Can you work these out from the model? Positions are in its coordinate system, mm. A direction names the side the tool comes from. Give positions to 0.01 mm unless a question says otherwise; leave off trailing zeros. Write each loop counter-clockwise with the first axis right and the second up, starting at its lowest first coordinate (ties: lowest second). Pieces come first, ordered by that corner, then holes.
Autodesk Inventor part; units mm, degrees
ref_plane "Work Plane1" through (0, 0, -15) normal (0, 0, 1) x (1, 0, 0)
ref_plane "YZ Plane" through (0, 0, 0) normal (1, 0, 0) x (0, 1, 0)
ref_plane "XZ Plane" through (0, 0, 0) normal (0, 1, 0) x (-1, 0, 0)
sketch "Sketch1" plane through (0, 0, 0) normal (0, 0, 1) x (1, 0, 0)
  line L0 (0, 0) -> (25, 0)
  line L1 (25, 0) -> (25, 40)
  line L2 (25, 40) -> (0, 40)
  line L3 (0, 40) -> (0, 0)
  dimension "d1" = 25
  dimension "d2" = 40
  dimension "d3" = 25
extrude "Extrusion1" add sketch "Sketch1" against normal blind 30
sketch "Sketch2" plane through (25, 0, 0) normal (1, 0, 0) x (0, 0, -1)
  line L0 (0, 0) -> (30, 0)
  circle A0 centre (15, 6.56) radius 2.46
extrude "Extrusion2" cut sketch "Sketch2" against normal blind 30
sketch "Sketch3" plane through (0, 0, 0) normal (-1, 0, 0) x (0, 0, 1)
  line L0 (0, 0) -> (-30, 0)
  line L1 (-25.05, 0) -> (-4.95, 0)
  line L2 (-4.95, 0) -> (-4.95, 33.12)
  line L3 (-4.95, 33.12) -> (-25.05, 33.12)
  line L4 (-25.05, 33.12) -> (-25.05, 0)
  dimension "d11" = 20.1
extrude "Extrusion3" cut sketch "Sketch3" against normal blind 20
sketch "Sketch4" plane through (0, 0, 0) normal (0, -1, 0) x (1, 0, 0)
  line L0 (20, -4.95) -> (20, -25.05)
  line L1 (20, -15) -> (25, -15)
  line L2 (25, 0) -> (25, -30)
  line L3 (20, -8.025) -> (25, -8.025)
  line L4 (25, -8.025) -> (25, -21.975)
  line L5 (25, -21.975) -> (20, -21.975)
  line L6 (20, -21.975) -> (20, -8.025)
  line L7 (20, -8.025) -> (25, -21.975) construction
  line L8 (25, -8.025) -> (20, -21.975) construction
  line L9 (25, -12.54) -> (25, -17.46)
  point P0 (0, 0)
  point P1 (22.5, -15)
  dimension "d14" = 13.95
extrude "Extrusion4" add sketch "Sketch4" along normal blind 15
sketch "Sketch5" plane through (20, 0, 0) normal (-1, 0, 0) x (0, 0, 1)
  circle A0 centre (-15, 6.56) radius 2.46
  circle A1 centre (-15, 6.56) radius 4.7025
  circle A2 centre (-15, 6.56) radius 2.46
  circle A3 centre (-15, 6.56) radius 2.46
  point P0 (0, 0)
  dimension "d17" = 9.405
extrude "Extrusion5" cut sketch "Sketch5" against normal blind 2.1
sketch "Sketch6" plane through (25, 0, 0) normal (1, 0, 0) x (0, 0, -1)
  circle A0 centre (15, 6.56) radius 4.7025
  line L0 (15, 6.56) -> (15, 23.56)
  circle A1 centre (15, 23.56) radius 2.46
  point P0 (0, 0)
  dimension "d20" = 17
  dimension "d21" = 4.92
extrude "Extrusion6" cut sketch "Sketch6" against normal blind 10 contours A1
sketch "Sketch7" plane through (20, 0, 0) normal (-1, 0, 0) x (0, 0, 1)
  circle A0 centre (-15, 23.56) radius 2.46
  circle A1 centre (-15, 23.56) radius 4.7025
  point P0 (0, 0)
  dimension "d24" = 9.405
extrude "Extrusion7" cut sketch "Sketch7" against normal blind 2.1
sketch "Sketch9" plane through (25, 0, 0) normal (1, 0, 0) x (0, 0, -1)
  circle A0 centre (15, 6.56) radius 2.46
  circle A1 centre (15, 6.56) radius 2.46
  circle A2 centre (15, 23.56) radius 2.46
  circle A3 centre (15, 23.56) radius 2.46
  line L0 (30, 40) -> (30, 0)
  line L1 (30, 0) -> (30, 40)
  line L2 (30, 40) -> (0, 40)
  line L3 (0, 40) -> (0, 0)
  line L4 (0, 0) -> (8.025, 0)
  line L5 (21.975, 0) -> (21.975, -15)
  line L6 (21.975, -15) -> (8.025, -15)
  line L7 (8.025, -15) -> (8.025, 0)
  line L8 (0, 0) -> (8.025, 0)
  line L9 (21.975, 0) -> (30, 0)
extrude "Extrusion8" add sketch "Sketch9" along normal blind 5
sketch "Sketch10" plane through (0, 40, 0) normal (0, 1, 0) x (1, 0, 0)
  line L0 (0, 30) -> (30, 30)
  line L1 (30, 0) -> (0, 0)
  line L2 (0, 30) -> (30, 30)
  line L3 (30, 30) -> (30, 0)
  line L4 (30, 0) -> (0, 0)
  line L5 (0, 0) -> (0, 30)
extrude "Extrusion9" add sketch "Sketch10" along normal blind 30
sketch "Sketch12" plane through (30, 0, 0) normal (1, 0, 0) x (0, 0, -1)
  circle A0 centre (15, 6.56) radius 2.46
  line L0 (15, 6.56) -> (15, 15.06)
  circle A1 centre (15, 15.06) radius 2.525
  point P0 (0, 0)
  dimension "d31" = 8.5
  dimension "d33" = 5.05
extrude "Extrusion10" cut sketch "Sketch12" against normal blind 30 contours A1
sketch "Sketch15" plane through (0, 0, -25.05) normal (-1, 0, 0) x (0, 0, 1)
  line L0 (0, 33.12) -> (20.1, 33.12)
  line L1 (20.1, 33.12) -> (20.1, 0)
  line L2 (0, 33.12) -> (20.1, 33.12)
  line L3 (20.1, 33.12) -> (20.1, 31.1)
  line L4 (20.1, 31.1) -> (0, 31.1)
  line L5 (0, 31.1) -> (0, 33.12)
  point P0 (25.05, 0)
  dimension "d57" = 2.02
extrude "Extrusion13" add sketch "Sketch15" against normal blind 20
sketch "Sketch17" plane through (0, 0, 0) normal (0, 0, 1) x (1, 0, 0)
  line L0 (0, 70) -> (30, 70)
  line L1 (30, 70) -> (50.0622, 90.0622)
  line L2 (30, 70) -> (80, 70) construction
  line L3 (11.9522, 97.2454) -> (0, 85.2932)
  line L4 (0, 70) -> (0, 85.2932)
  line L5 (0, 70) -> (0, 0)
  line L6 (0, 70) -> (30, 70)
  line L7 (10.923, 112.2849) -> (0, 120.567)
  line L8 (50.0622, 105.3553) -> (50.0622, 120.567)
  line L9 (50.0622, 105.3553) -> (50.0622, 90.0622)
  arc A0 (11.9522, 97.2454) -> (10.923, 112.2849) centre (4.8811, 104.3165) ccw
  line L10 (0, 150.567) -> (30, 150.567)
  line L11 (30, 150.567) -> (50.0622, 120.567)
  line L12 (5, 147.567) -> (0, 150.567)
  line L13 (5, 123.567) -> (0, 120.567)
  line L14 (5, 123.567) -> (10, 135.567)
  line L15 (10, 135.567) -> (5, 147.567)
  dimension "d61" = 45
  dimension "d62" = 32.0271
  dimension "d72" = 10
extrude "Extrusion14" add sketch "Sketch17" against normal blind 30
sketch "Sketch22" plane through (0, 0, 0) normal (0, 0, 1) x (1, 0, 0)
  line L0 (30, 0) -> (30, 70)
  line L1 (50.0622, 120.567) -> (50.0622, 90.0622)
  line L2 (30, 70) -> (50.0622, 90.0622)
  line L3 (50.0622, 90.0622) -> (50.0622, 120.567)
  line L4 (50.0622, 120.567) -> (30, 150.567)
  line L5 (50.0622, 120.567) -> (30, 150.567)
  line L6 (30, 150.567) -> (0, 150.567)
  line L7 (30, 150.567) -> (0, 150.567)
  line L8 (0, 150.567) -> (5, 147.567)
  line L9 (0, 150.567) -> (5, 147.567)
  line L10 (5, 147.567) -> (10, 135.567)
  line L11 (5, 147.567) -> (10, 135.567)
  line L12 (5, 123.567) -> (10, 135.567)
  line L13 (10, 135.567) -> (5, 123.567)
  line L14 (5, 123.567) -> (0, 120.567)
  line L15 (5, 123.567) -> (0, 120.567)
  line L16 (10.923, 112.2849) -> (0, 120.567)
  line L17 (0, 120.567) -> (10.923, 112.2849)
  line L18 (0, 85.2932) -> (11.9522, 97.2454)
  line L19 (11.9522, 97.2454) -> (0, 85.2932)
  line L20 (0, 85.2932) -> (0, 55.2932)
  line L21 (0, 0) -> (0, 85.2932)
  line L22 (0, 55.2932) -> (30, 55.2932)
  line L23 (30, 55.2932) -> (30, 70)
  arc A0 (11.9522, 97.2454) -> (10.923, 112.2849) centre (4.8811, 104.3165) ccw
  arc A1 (11.9522, 97.2454) -> (10.923, 112.2849) centre (4.8811, 104.3165) ccw
  dimension "d87" = 30
extrude "Extrusion15" add sketch "Sketch22" along normal blind 45
ref_plane "Work Plane1" through (0, 0, -15) normal (0, 0, 1) x (1, 0, 0)
mirror "Mirror1" about plane through (0, 0, -15) normal (0, 0, 1) of "Extrusion15"
properties part number "rec_c_24mm_x_120mm"
1) Suppose I cut it at C-C on z = -15. State how many separate pieces and enclosed holes the cut face has, plus the area to 3 significant figures.
Values follow:
separate pieces: 4
enclosed holes: 0
area: 4,470 mm2
2) If we mould it in two halves opening along Z, with no side actions, what happens to faces 6 (the face through (21.035, 7.973, -10.515)), 7 (the face through (25, 104, 45)), 8 (the face through (14.865, 104.88, -14.16)), 9 (the face through (22.1, 21.5, -13))? For each: +Z half, -Z half, draft (parallel to the pull), parting line (faces both ways), or undercut.
Values follow:
face 6: undercut
face 7: +Z half
face 8: draft
face 9: undercut
3) For faces 1 (the face through (15, 28, 0)), 2 (the face through (20, 8, -20)), 3 (the face through (30, 47, -14)), 4 (the face through (7.535, 129.651, -14.16)), 5 (the face through (21.035, 27.525, -12.472)), which set-ups out of +Z, -Z, +X, -X, +Y, -Y let a thin tool reach every point of the face, with its end or its side?
Values follow:
face 1: +Z, +X, -X, -Y
face 2: -X, -Y
face 3: +Z, -Z, +X, -Y
face 4: +Z, -Z, -X
face 5: -X
4) Please list where these lines run through material, in increasing order: L1, parallel to Y at x = 21.2, z = -15 (1 decimal); L2, parallel to Y at x = 24, z = -15 (3 decimals); L3, parallel to Z at x = 21, y = 23.
Values follow:
L1: y = -15 to 1.9, 11.3 to 12.5, 17.6 to 18.9, 28.3 to 150.6
L2: y = -15 to 4.1, 9.02 to 12.535, 17.585 to 21.1, 26.02 to 150.567
L3: z = -30 to -19.67, -10.33 to 0
5) Suppose I cut it at B-B on z = -62. Write out the boundary of the cut face in (x, y), plus the area to 3 significant figures.
Values follow:
outline: (0, 55.29) - (30, 55.29) - (30, 70) - (50.06, 90.06) - (50.06, 120.57) - (30, 150.57) - (0, 150.57) - (5, 147.57) - (10, 135.57) - (5, 123.57) - (0, 120.57) - (10.92, 112.28) arc R10 cw to (11.95, 97.25) - (0, 85.29) - close
area: 3,450 mm2
6) Suppose I cut it at A-A on y = 15.06. Write out the boundary of the cut face in (x, z) (3 decimals).
Values follow:
outline: (0, -30) - (30, -30) - (30, -17.525) - (20, -17.525) - (20, -25.05) - (0, -25.05) - close; (0, -4.95) - (20, -4.95) - (20, -12.475) - (30, -12.475) - (30, 0) - (0, 0) - close
7) For pin 1 Ø6 at (y, z) = (130.5, -4.5) entering from -X; pin 2 Ø6.5 at (y, z) = (15.06, -15) entering from +X; pin 3 Ø8 at (x, y) = (27, -9) entering from -Z (3 decimals), each with a flat end and sliding along its axis, tell me the tip position at first contact or that it passes through.
Values follow:
pin 1: stops at x = 6.64
pin 2: stops at x = 30
pin 3: stops at z = -21.975
8) Suppose I cut it at D-D on y = 33.5. Write out the boundary of the cut face in (x, z), plus the area to 3 significant figures.
Values follow:
outline: (0, -30) - (30, -30) - (30, 0) - (0, 0) - close
area: 900 mm2
